Verification items for the finished model (mm, model axes). Face numbers are marked on the shaded views. Coordinates: 2 decimals unless noted, no trailing zeros. Loops run counter-clockwise (first coordinate to the right, second up) from the corner with the lowest first, then second, coordinate; pieces in that order, holes last. Notation, with made-up numbers: (-20, 67) -> (13, 67) arc R29 cw to (13, 88) -> close; hole circle Ø8 at (40.5, 3.25). An arc over 180 degrees is marked (long way). Answer as a JSON object with one key per item and string values. Group by question number.
Q1. Cross-section at C-C on y = 14. Record the boundary of the cut face in (x, z), and give its area (3 significant figures).
Q2. Gauge pin test, flat ends, axial feed: pin 1 Ø3 at (x, y) = (11.5, 10.5) entering from -Z; pin 2 Ø1.5 at (x, y) = (-1, 3) entering from +Z; pin 3 Ø1.5 at (x, z) = (-8, 6) entering from +Y; pin 4 Ø10 at (y, z) = (-3, 13) entering from -X. Record the tip position at first contact, or that the pin passes through.
Q3. Release check for a two-part mould opening along Y. For the marked faces 1, 2 and 3 record: released by +Y, released by -Y, zero draft, split by the parting line, or undercut.
Q4. Cross-section at A-A on y = 0.5. Record the boundary of the cut face in (x, z), and give its area (3 significant figures).
Q5. Cross-section at B-B on y = -6.5. Record the boundary of the cut face in (x, z).
Q6. Scan lines: L1, parallel to Y at x = -2, z = 10; L2, parallel to Z at x = -4.5, y = 11.5; L3, parallel to Y at x = 2, z = 9.25. Record each from-to range of solid material in increasing order.
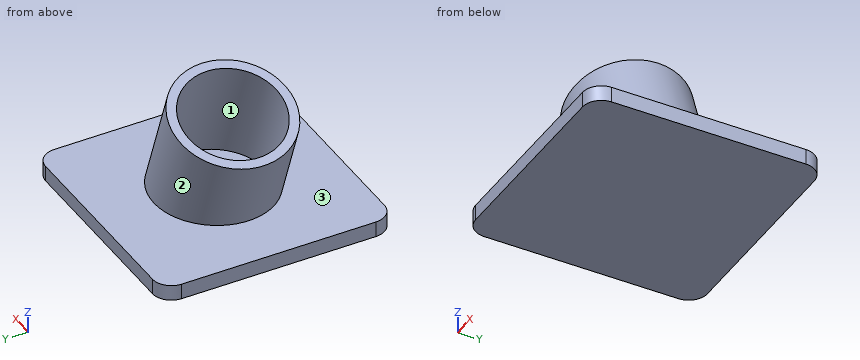
```python
from build123d import *

# Parameters (mm, degrees)
EXTRUDE_1_DEPTH     = 2.5
EXTRUDE_3_REACH     = 31.489
SKETCH_6_R          = 9.5
EXTRUDE_START       = 10
SKETCH_12_R         = 9.5
EXTRUDE_4_DEPTH     = 10
CUT_EXTRUDE_4_REACH = 37.632
SKETCH_13_R         = 8


with BuildPart() as part:
    # 草圖1 → 填料-伸長1 (new body)
    with BuildSketch(Plane.XY):
        with BuildLine():
            Line((-15.5, -18.5), (15.5, -18.5))
            ThreePointArc((15.5, -18.5), (17.621320344, -17.621320344), (18.5, -15.5))
            Line((18.5, -15.5), (18.5, 15.5))
            ThreePointArc((18.5, 15.5), (17.621320344, 17.621320344), (15.5, 18.5))
            Line((15.5, 18.5), (-15.5, 18.5))
            ThreePointArc((-15.5, 18.5), (-17.621320344, 17.621320344), (-18.5, 15.5))
            Line((-18.5, 15.5), (-18.5, -15.5))
            ThreePointArc((-18.5, -15.5), (-17.621320344, -17.621320344), (-15.5, -18.5))
        make_face()
    extrude(amount=EXTRUDE_1_DEPTH)

    # 填料-伸長3: up to this plane
    extrude_3_end = Plane(origin=(-15.5, 15.5, 2.5), z_dir=(0, 0, -1))
    # 草圖6 → 填料-伸長3 (add, up to the surface)
    with BuildSketch(Plane(origin=(-2.967573413, 0, 8.153340943), x_dir=(0, -1, 0), z_dir=(-0.34202014332566943, 0, 0.9396926207859081)), mode=Mode.PRIVATE) as extrude_3_sk1:
        with Locations(Location((0, 1.280349356, 0), (0, 0, 90))):
            Circle(SKETCH_6_R)
    extrude_3_tool1 = split(extrude(extrude_3_sk1.sketch, amount=-EXTRUDE_3_REACH, mode=Mode.PRIVATE), bisect_by=extrude_3_end, keep=Keep.BOTH, mode=Mode.PRIVATE)
    add(extrude_3_tool1.solids().sort_by_distance((-1.764439, 0, 8.591246))[0])

    # 草圖12 → 填料-伸長4 (add)
    with BuildSketch(Plane(origin=(-2.967573413, 0, 8.153340943), x_dir=(0.9396926207859082, 0, 0.3420201433256695), z_dir=(-0.3420201433256695, 0, 0.9396926207859082)).offset(EXTRUDE_START)):
        with Locations((1.280349356, 0)):
            Circle(SKETCH_12_R)
    extrude(amount=-EXTRUDE_4_DEPTH)

    # 除料-伸長4: up to this plane
    cut_extrude_4_end = Plane(origin=(-15.5, 15.5, 2.5), z_dir=(0, 0, -1))
    # 草圖13 → 除料-伸長4 (cut, up to the surface)
    with BuildSketch(Plane(origin=(-6.387774847, 0, 17.550267151), x_dir=(0.9396926207859082, 0, 0.3420201433256695), z_dir=(-0.3420201433256695, 0, 0.9396926207859082)), mode=Mode.PRIVATE) as cut_extrude_4_sk1:
        with Locations((1.280349356, 0)):
            Circle(SKETCH_13_R)
    cut_extrude_4_tool1 = split(extrude(cut_extrude_4_sk1.sketch, amount=-CUT_EXTRUDE_4_REACH, mode=Mode.PRIVATE), bisect_by=cut_extrude_4_end, keep=Keep.BOTH, mode=Mode.PRIVATE)
    add(cut_extrude_4_tool1.solids().sort_by_distance((-5.18464, 0, 17.988172))[0], mode=Mode.SUBTRACT)


solid = part.part
```
Computed values:
{
 "1": {"outline": "(-18.5, 0) -> (18.5, 0) -> (18.5, 2.5) -> (-18.5, 2.5) -> close", "area": "92.5 mm²"},
 "2": {"pin 1": "stops at z = 0", "pin 2": "stops at z = 2.5", "pin 3": "stops at y = 7.37", "pin 4": "stops at x = -14.11"},
 "3": {"face 1": "undercut", "face 2": "split by the parting line", "face 3": "zero draft"},
 "4": {"outline": "(-18.5, 0) -> (18.5, 0) -> (18.5, 2.5) -> (10.55, 2.5) -> (3.73, 21.23) -> (2.32, 20.72) -> (8.95, 2.5) -> (-8.04, 2.5) -> (-12.69, 15.26) -> (-14.1, 14.74) -> (-9.64, 2.5) -> (-18.5, 2.5) -> close", "area": "142 mm²"},
 "5": {"outline": "(-18.5, 0) -> (18.5, 0) -> (18.5, 2.5) -> (7.83, 2.5) -> (1.33, 20.36) -> (-0.8, 19.58) -> (5.42, 2.5) -> (-4.51, 2.5) -> (-9.57, 16.39) -> (-11.7, 15.62) -> (-6.92, 2.5) -> (-18.5, 2.5) -> close"},
 "6": {"L1": "y = -9.5 to -8, 8 to 9.5", "L2": "z = 0 to 2.5", "L3": "y = -8.72 to -7.06, 7.06 to 8.72"}
}
